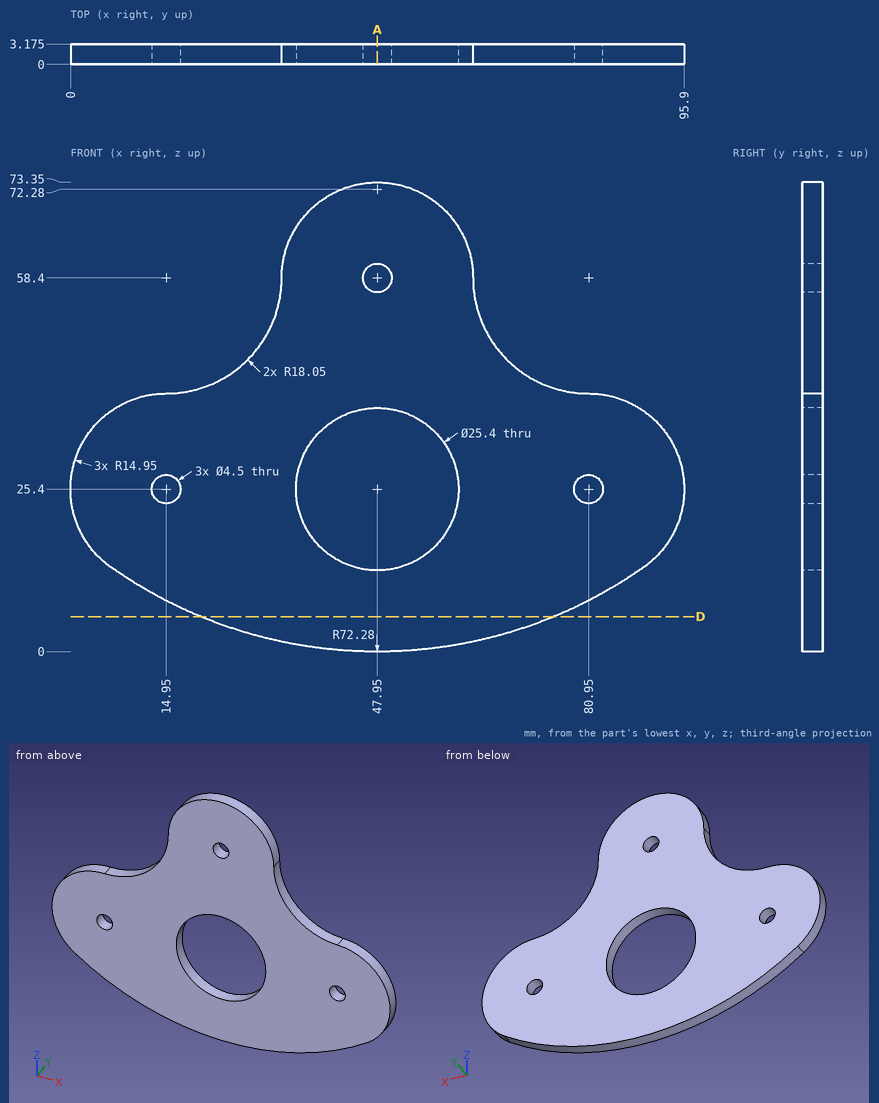
Check sheet for the drawn part. Datum: minimum x, y, z corner. Units: mm. Give positions to 0.01 mm unless a question says otherwise; leave off trailing zeros. Loops run counter-clockwise (first coordinate to the right, second up) from the corner with the lowest first, then second, coordinate; pieces in that order, holes last.
1) Depth check by flat-ended pin: pin 1 Ø7 at (x, z) = (80.95, 25.4) entering from -Y; pin 2 Ø1 at (x, y) = (14.5, 3) entering from +Z. Enter the tip coordinate at first touch or a pass-through.
2) Sectioned sample at D-D, the plane z = 5.5. Enter the section's corners in (x, y) (1 decimal).
3) Thickness scan on line 1 along Z through (x, y) = (80.95, 2); line 2 along X through (y, z) = (2.3, 20.5) (1 decimal). Record the ranges inside material, lowest first.
4) Sectioned sample at A-A, the plane x = 47.95. Count the separate pieces of the cut face and the enclosed holes in it, then the cut area to 3 significant figures.
Answers:
1. pin 1: stops at y = 0
1. pin 2: stops at z = 40.35
2. outline: (20.3, 0) - (75.6, 0) - (75.6, 3.2) - (20.3, 3.2) - close
3. line 1: z = 7.97 to 23.15, 27.65 to 40.35
3. line 2: x = 0.8 to 36.2, 59.7 to 95.1
4. separate pieces: 3
4. enclosed holes: 0
4. area: 138 mm2
